Autodesk Inventor part; units mm, degrees
ref_plane "YZ Plane" through (0, 0, 0) normal (1, 0, 0) x (0, 1, 0)
ref_plane "XZ Plane" through (0, 0, 0) normal (0, 1, 0) x (-1, 0, 0)
ref_plane "XY Plane" through (0, 0, 0) normal (0, 0, 1) x (1, 0, 0)
sketch "Sketch1" plane through (0, 0, 0) normal (0, 1, 0) x (-1, 0, 0)
  line L0 (9.075, 10.425) -> (-9.075, 10.425)
  line L1 (-10.075, 9.425) -> (-10.075, -9.425)
  line L2 (-9.075, -10.425) -> (9.075, -10.425)
  line L3 (10.075, -9.425) -> (10.075, 9.425)
  line L4 (10.075, 10.425) -> (-10.075, -10.425) construction
  line L5 (-10.075, 10.425) -> (10.075, -10.425) construction
  arc A0 (9.075, -10.425) -> (10.075, -9.425) centre (9.075, -9.425) ccw
  arc A1 (-10.075, -9.425) -> (-9.075, -10.425) centre (-9.075, -9.425) ccw
  arc A2 (-9.075, 10.425) -> (-10.075, 9.425) centre (-9.075, 9.425) ccw
  arc A3 (10.075, 9.425) -> (9.075, 10.425) centre (9.075, 9.425) ccw
  circle A4 centre (7.035, -7.385) radius 1.5
  line L6 (10.075, 0) -> (-10.075, 0) construction
  line L7 (0, -10.425) -> (0, 10.425) construction
  circle A5 centre (7.035, 7.385) radius 1.5
  circle A6 centre (-7.035, -7.385) radius 1.5
  circle A7 centre (-7.035, 7.385) radius 1.5
  point P0 (0, 0)
  dimension "d0" = 20.15
  dimension "d1" = 20.85
  dimension "d4" = 1
  dimension "d5" = 3
  dimension "d6" = 3.04
  dimension "d7" = 3.04
extrude "Extrusion2" add sketch "Sketch1" along normal blind 1.56
sketch "Sketch2" plane through (0, 1.56, 0) normal (0, 1, 0) x (1, 0, 0)
  line L0 (-4.2426, 0) -> (0, 4.2426)
  line L1 (0, 4.2426) -> (4.2426, 0)
  line L2 (4.2426, 0) -> (0, -4.2426)
  line L3 (0, -4.2426) -> (-4.2426, 0)
  line L4 (-3, 3) -> (3, -3) construction
  line L5 (3, 3) -> (-3, -3) construction
  point P0 (0, 0)
  dimension "d10" = 6
  dimension "d11" = 6
extrude "Extrusion3" add sketch "Sketch2" along normal blind 3.5
sketch "Sketch3" plane through (0, 1.56, 0) normal (0, 1, 0) x (1, 0, 0)
  line L0 (4, -10.425) -> (-4, -10.425)
  line L1 (-4, -10.425) -> (-4, -7.895)
  line L2 (-4, -7.895) -> (4, -7.895)
  line L3 (4, -7.895) -> (4, -10.425)
  line L4 (-9.075, -10.425) -> (9.075, -10.425) construction
  line L5 (0, -10.425) -> (0, 10.4665) construction
  point P0 (0, 0)
  dimension "d14" = 8
  dimension "d15" = 2.53
extrude "Extrusion4" add sketch "Sketch3" along normal blind 4.2
sketch "Sketch4" plane through (0, 0, 0) normal (0, -1, 0) x (1, 0, 0)
  line L0 (2.9048, 3.5) -> (5.9048, 3.5)
  line L1 (5.9048, 3.5) -> (5.9048, -3.5)
  line L2 (5.9048, -3.5) -> (2.9048, -3.5)
  line L3 (2.9048, -3.5) -> (2.9048, 3.5)
  line L4 (-14.105, 0) -> (14.105, 0)
  point P0 (0, 0)
  point P1 (2.9048, 0)
  dimension "d18" = 3
  dimension "d19" = 7
extrude "Extrusion5" add sketch "Sketch4" along normal blind 3
sketch "Sketch5" plane through (0, 5.06, 0) normal (0, 1, 0) x (1, 0, 0)
  circle A0 centre (0, 0) radius 1.75
  dimension "d22" = 3.5
extrude "Extrusion6" add sketch "Sketch5" along normal blind 2.54
equation "\"d7\" = d6"
properties part number "board_blueprint"
Work out the finished part from the listing and answer in its coordinate system (mm). A direction names the side the tool comes from. Give positions to 0.01 mm unless a question says otherwise; leave off trailing zeros. Loops run counter-clockwise (first coordinate to the right, second up) from the corner with the lowest first, then second, coordinate; pieces in that order, holes last. Notation, with made-up numbers: (-13, 20.5) -> (26, 20.5) arc R28 ccw to (26, 57.5) -> close; hole circle Ø5 at (53, 33). An arc over 180 degrees is marked (long way). Use CSV: the item, a comma, the result in double quotes.
1. The part is cut by section A-A (y = 3.25). Write down the section's boundary in (x, z) (3 decimals).
Found:
outline,"(-4.243, 0) -> (0, -4.243) -> (4.243, 0) -> (0, 4.243) -> close; (-4, 7.895) -> (4, 7.895) -> (4, 10.425) -> (-4, 10.425) -> close"
2. The mould has two halves that part along Z. Classify faces 5 (the flat face through (2.09, 3.29, -2.15)), 6 (the flat face through (0, 5.76, 9)), 7 (the flat face through (-2, 5.06, 0)), 8 (the cylindrical face through (-8.466, 0.769, 6.934)): +Z half, -Z half, draft (parallel to the pull), parting line (faces both ways), or undercut.
Found:
face 5,"-Z half"
face 6,"draft"
face 7,"undercut"
face 8,"undercut"
3. Flat-ended cylindrical pins translate along their axes: pin 1 Ø5 at (x, z) = (7.035, 7.385) entering from +Y; pin 2 Ø4.5 at (x, y) = (0, 4) entering from -Z; pin 3 Ø2 at (x, z) = (1.5, 9) entering from +Y. Find the tip coordinate at first contact, or state that the pin passes through.
Found:
pin 1,"y = 1.56"
pin 2,"z = -4.24"
pin 3,"y = 5.76"
4. A tool of negligible diameter and unlimited length cuts with its end or side. For faces 1 (the cylindrical face through (-7.727, 0.769, -6.054)), 2 (the flat face through (0, 4, 7.895)), 3 (the flat face through (-2.09, 3.29, 2.15)), 4 (the flat face through (-4, 4, 9)), from which of +Z, -Z, +X, -X, +Y, -Y can it reach the whole face along a straight path? Write none if from no direction.
Found:
face 1,"+Y, -Y"
face 2,"+X, -X, +Y"
face 3,"-X, +Y"
face 4,"+Z, -X, +Y"
5. The part is cut by section B-B (x = -7). Write down the section's boundary in (y, z) (3 decimals), then the cut area to 3 significant figures.
Found:
outline,"(0, -10.425) -> (1.56, -10.425) -> (1.56, -8.885) -> (0, -8.885) -> close; (0, -5.885) -> (1.56, -5.885) -> (1.56, 5.885) -> (0, 5.885) -> close; (0, 8.885) -> (1.56, 8.885) -> (1.56, 10.425) -> (0, 10.425) -> close"
area,"23.2 mm^2"
6. The part is cut by section C-C (x = 5). Write down the section's boundary in (y, z) (3 decimals), then the cut area to 3 significant figures.
Found:
outline,"(-3, -3.5) -> (0, -3.5) -> (0, -10.425) -> (1.56, -10.425) -> (1.56, 10.425) -> (0, 10.425) -> (0, 3.5) -> (-3, 3.5) -> close"
area,"53.5 mm^2"
7. Straight lines are drawn through the part: line 1 (Z direction, x = 7, y = 1) (3 decimals); line 2 (Y direction, x = 7.75, z = 1); line 3 (Z direction, x = -3, y = 5.25) (3 decimals). For each, find the intervals that lie inside material, in ascending order.
Found:
line 1,"-10.425 to -8.885, -5.885 to 5.885, 8.885 to 10.425"
line 2,"0 to 1.56"
line 3,"7.895 to 10.425"
8. The part is cut by section D-D (z = -2.5). Write down the section's boundary in (x, y) (3 decimals).
Found:
outline,"(-10.075, 0) -> (2.905, 0) -> (2.905, -3) -> (5.905, -3) -> (5.905, 0) -> (10.075, 0) -> (10.075, 1.56) -> (1.743, 1.56) -> (1.743, 5.06) -> (-1.743, 5.06) -> (-1.743, 1.56) -> (-10.075, 1.56) -> close"
